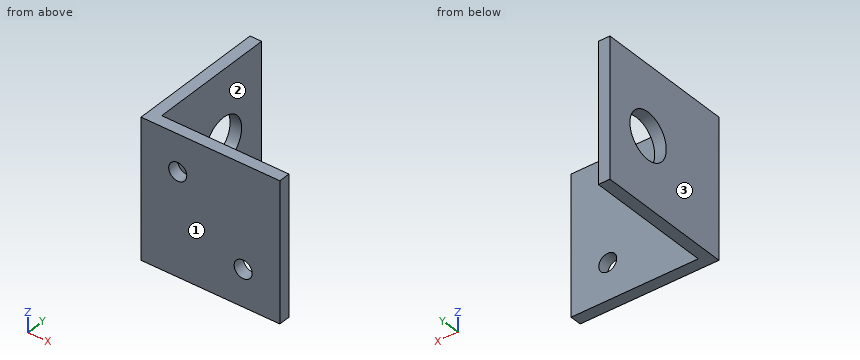
```python
from build123d import *

# Parameters (mm, degrees)
EXTRUDE_THIN1_DEPTH = 38.1
SKETCH2_R           = 6.35
CUT_EXTRUDE1_DEPTH  = 39.1
SKETCH3_R           = 2.4765
CUT_EXTRUDE2_DEPTH  = 39.1


with BuildPart() as part:
    # Sketch1 → Extrude-Thin1 (new body)
    with BuildSketch(Plane.XY):
        Polygon((0, 38.1), (0, 0), (38.1, 0), (38.1, 3.175), (3.175, 3.175), (3.175, 38.1), align=None)
    extrude(amount=EXTRUDE_THIN1_DEPTH)

    # Sketch2 → Cut-Extrude1 (cut, through all)
    with BuildSketch(Plane.ZY):
        with Locations((19.05, 24.765)):
            Circle(SKETCH2_R)
    extrude(amount=-CUT_EXTRUDE1_DEPTH, mode=Mode.SUBTRACT)

    # Sketch3 → Cut-Extrude2 (cut, through all)
    with BuildSketch(Plane.XZ):
        with Locations((28.030256121, 10.069743879)):
            Circle(SKETCH3_R)
        with Locations((10.069743879, 28.030256121)):
            Circle(SKETCH3_R)
    extrude(amount=-CUT_EXTRUDE2_DEPTH, mode=Mode.SUBTRACT)


solid = part.part
```
Can you work these out from the model? Positions are in its coordinate system, mm. Face numbers are marked on the shaded views. Coordinates: 2 decimals unless noted, no trailing zeros. Order: outer loops, then holes, each group sorted by start corner. A loop starts at its lowest first (then second) coordinate and runs counter-clockwise, first axis right, second up.
1. If we section it at A-A (z = 19.05): Please give me the cut outline in (x, y) (3 decimals), then the cut area to 3 significant figures.
2. I need wall thicknesses on line 1 (Y direction, x = 2.2, z = 19.05) (3 decimals); line 2 (X direction, y = 14, z = 32) (3 decimals). Which ranges of each line are inside material? Lowest first, please.
3. I'm going to push flat-ended pins straight in: pin 1 (4 mm diameter, centred on x = 10.07, z = 28.03, fed in from -Y); pin 2 (1.5 mm diameter, centred on y = 7.5, z = 13, fed in from +X) (3 decimals); pin 3 (5 mm diameter, centred on x = 16, z = 32.5, fed in from +Y) (3 decimals). Where does each tip first touch, or does it pass through?
4. Thinking about a two-plate mould opening in X: for the marked faces 1, 2 and 3, which applies, +X half, -X half, draft (parallel to the pull), parting line (faces both ways), or undercut?
5. If we section it at D-D (z = 27): Please give me the cut outline in (x, y) (3 decimals), then the cut area to 3 significant figures.
6. If we section it at B-B (x = 18.5): Please give me the cut outline in (y, z) (3 decimals), then the cut area to 3 significant figures.
7. If we section it at C-C (z = 5): Please give me the cut outline in (x, y) (3 decimals), then the cut area to 3 significant figures.
Entries:
1. outline: (0, 0) - (38.1, 0) - (38.1, 3.175) - (3.175, 3.175) - (3.175, 18.415) - (0, 18.415) - close; (0, 31.115) - (3.175, 31.115) - (3.175, 38.1) - (0, 38.1) - close
1. area: 192 mm2
2. line 1: y = 0 to 18.415, 31.115 to 38.1
2. line 2: x = 0 to 3.175
3. pin 1: passes through
3. pin 2: stops at x = 3.175
3. pin 3: stops at y = 3.175
4. face 1: draft
4. face 2: +X half
4. face 3: -X half
5. outline: (0, 0) - (7.818, 0) - (7.818, 3.175) - (3.175, 3.175) - (3.175, 38.1) - (0, 38.1) - close; (12.322, 0) - (38.1, 0) - (38.1, 3.175) - (12.322, 3.175) - close
5. area: 218 mm2
6. outline: (0, 0) - (3.175, 0) - (3.175, 38.1) - (0, 38.1) - close
6. area: 121 mm2
7. outline: (0, 0) - (38.1, 0) - (38.1, 3.175) - (3.175, 3.175) - (3.175, 38.1) - (0, 38.1) - close
7. area: 232 mm2
